```python
from build123d import *

# Parameters (mm, degrees)
F0_R     = 2
F1_DEPTH = 5


with BuildPart() as f1:
    # F0 (on Top) → F1 (new body)
    with BuildSketch(Plane.XY):
        with BuildLine():
            ThreePointArc((-3, 2.645751), (0, 4), (3, 2.645751))
            Line((3, 2.645751), (3, 13.645751))
            Line((3, 13.645751), (-3, 8.354249))
            Line((-3, 8.354249), (-3, 2.645751))
        make_face()
        with BuildLine():
            ThreePointArc((0, -4), (2.828427, -2.828427), (4, 0))
            ThreePointArc((4, 0), (3.741657, 1.414214), (3, 2.645751))
            ThreePointArc((3, 2.645751), (0, 4), (-3, 2.645751))
            ThreePointArc((-3, 2.645751), (-3.963267, -0.540843), (-2.18141, -3.352827))
            ThreePointArc((-2.18141, -3.352827), (-1.137693, -3.834795), (0, -4))
        make_face()
        Circle(F0_R, mode=Mode.SUBTRACT)
        with BuildLine():
            ThreePointArc((3.779688, -23.968328), (-0.100807, -14.360962), (0, -4))
            ThreePointArc((0, -4), (-1.137693, -3.834795), (-2.18141, -3.352827))
            ThreePointArc((-2.18141, -3.352827), (-2.104688, -14.500237), (3.779688, -23.968328))
        make_face()
    extrude(amount=F1_DEPTH)


solid = f1.part
```
Geometry check sheet. Reference: the model listing, model coordinates, mm. A direction names the side the tool comes from. Round coordinates to 2 decimals unless told otherwise and drop trailing zeros. Order: outer loops, then holes, each group sorted by start corner. A loop starts at its lowest first (then second) coordinate and runs counter-clockwise, first axis right, second up. Notation, with made-up numbers: (-32.5, 82) - (9.5, 82) arc R36 ccw to (9.5, 121) - close; hole circle Ø5 at (34.25, -26.75). An arc over 180 degrees is marked (long way). Use a Markdown table: item, result. Add a question column.
(1) Sectioned sample at A-A, the plane z = 3.7. Enter the section's corners in (x, y), and give its area (3 significant figures).
(2) Depth check by flat-ended pin: pin 1 (2.5 mm diameter, centred on y = 4, z = 1.5, fed in from -X); pin 2 (1.5 mm diameter, centred on y = 9.5, z = 3, fed in from +X); pin 3 (3 mm diameter, centred on x = 0, y = 0, fed in from -Z); pin 4 (1 mm diameter, centred on x = -2.5, z = 2.5, fed in from +Y). Enter the tip coordinate at first touch or a pass-through.
(3) Release check for a two-part mould opening along X. For faces 4 (the flat face through (-3, -1, 5)), 5 (the cylindrical face through (0, -2, 2)), 6 (the flat face through (0, 11, 2)) record: pulls with the +X half, pulls with the -X half, needs draft (parallel to the pull), parting line crosses it, or undercut.
(4) Material ranges on line 1 along X through (y, z) = (-1, 1.3); line 2 along X through (y, z) = (10.5, 2.3); line 3 along Y through (x, z) = (1.5, 3.45), recorded low to high. Write a range as [from, to].
(5) Sectioned sample at D-D, the plane y = -15.5. Enter the section's corners in (x, z), and give its area (3 significant figures).
(6) Tool access check on faces 1 (the flat face through (-3, 6, 2)), 2 (the flat face through (3, 8, 2)), 3 (the flat face through (-3, -1, 0)). Record the directions out of +Z, -Z, +X, -X, +Y, -Y that give a thin tool (end or side, any length) a straight path to the whole face; none if there is none.
(7) Sectioned sample at C-C, the plane y = 3.5. Enter the section's corners in (x, z).
(8) Sectioned sample at B-B, the plane x = 1. Enter the section's corners in (y, z), and give its area (3 significant figures).
Answers below:
| question | item | result |
|---|---|---|
| 1 | outline | (-3, 2.65) arc R4 ccw to (-2.18, -3.35) arc R20.56 ccw to (3.78, -23.97) arc R26.5 cw to (0, -4) arc R4 ccw to (4, 0) arc R4 ccw to (3, 2.65) - (3, 13.65) - (-3, 8.35) - close; hole circle Ø4 at (0, 0) |
| 1 | area | 119 mm² |
| 2 | pin 1 | x = -3 |
| 2 | pin 2 | x = 3 |
| 2 | pin 3 | through |
| 2 | pin 4 | y = 9.24 |
| 3 | face 4 | needs draft |
| 3 | face 5 | undercut |
| 3 | face 6 | pulls with the -X half |
| 4 | line 1 | [-3.87, -1.73], [1.73, 3.87] |
| 4 | line 2 | [-0.57, 3] |
| 4 | line 3 | [-21.52, -19.68], [-3.71, -1.32], [1.32, 12.32] |
| 5 | outline | (-1.79, 0) - (0.14, 0) - (0.14, 5) - (-1.79, 5) - close |
| 5 | area | 9.64 mm² |
| 6 | face 1 | +Z, -Z, -X, +Y |
| 6 | face 2 | +Z, -Z, +X, +Y |
| 6 | face 3 | -Z, +X, -X, +Y, -Y |
| 7 | outline | (-3, 0) - (3, 0) - (3, 5) - (-3, 5) - close |
| 8 | outline | (-20.86, 0) - (-18.4, 0) - (-18.4, 5) - (-20.86, 5) - close; (-3.87, 0) - (-1.73, 0) - (-1.73, 5) - (-3.87, 5) - close; (1.73, 0) - (11.88, 0) - (11.88, 5) - (1.73, 5) - close |
| 8 | area | 73.7 mm² |
